from build123d import *

# Parameters (mm, degrees)
F0_W           = 127
F0_H           = 19.05
F1_DEPTH       = 88.9
F2_R           = 3.937
F2_R_2         = 2.413
F3_DEPTH       = 19.05
F5_D           = 6.35
F5_CBORE_D     = 11.176
F5_CBORE_DEPTH = 6.35
F7_DEPTH       = 19.051
F8_R           = 3.048


with BuildPart() as f1:
    # F0 (on Front) → F1 (new body)
    with BuildSketch(Plane.XZ):
        Rectangle(F0_W, F0_H)
    extrude(amount=-F1_DEPTH)

    # F2 (on face) → F3 (cut, through all)
    with BuildSketch(Plane.XY.offset(9.525)):
        with Locations((-53.975, 73.025)):
            Circle(F2_R)
        with Locations((-53.975, 9.525)):
            Circle(F2_R)
        with Locations((53.975, 9.525)):
            Circle(F2_R)
        with Locations((53.975, 73.025)):
            Circle(F2_R)
        with Locations((-6.35, 38.1)):
            Circle(F2_R_2)
        with Locations((12.7, 38.1)):
            Circle(F2_R_2)
        with Locations((12.7, 12.7)):
            Circle(F2_R_2)
        with Locations((-6.35, 12.7)):
            Circle(F2_R_2)
    extrude(amount=-F3_DEPTH, mode=Mode.SUBTRACT)

    # F5 (through all)
    with Locations(Plane(origin=(0, 0, -9.525), x_dir=(1, 0, 0), z_dir=(0, 0, -1))):
        with Locations((25.4, -69.85), (25.4, -44.45), (-41.275, -31.75), (-41.275, -6.35)):
            CounterBoreHole(F5_D / 2, F5_CBORE_D / 2, F5_CBORE_DEPTH)

    # F6 (on face) → F7 (cut, through all)
    with BuildSketch(Plane(origin=(0, 0, -9.525), x_dir=(1, 0, 0), z_dir=(0, 0, -1))):
        with BuildLine():
            ThreePointArc((63.5, -81.5884231275), (0, -88.9), (-63.5, -81.5884231275))
            Line((-63.5, -81.5884231275), (-63.5, -94.2089855671))
            Line((-63.5, -94.2089855671), (63.5, -94.2089855671))
            Line((63.5, -94.2089855671), (63.5, -81.5884231275))
        make_face()
    extrude(amount=-F7_DEPTH, mode=Mode.SUBTRACT)

    # F8
    f8_edges = [f1.edges().sort_by_distance(p)[0] for p in [
        (63.5, 81.588423, 0),
        (63.5, 0, 0),
        (-63.5, 81.588423, 0),
        (-63.5, 0, 0),
    ]]
    fillet(f8_edges, radius=F8_R)


solid = f1.part
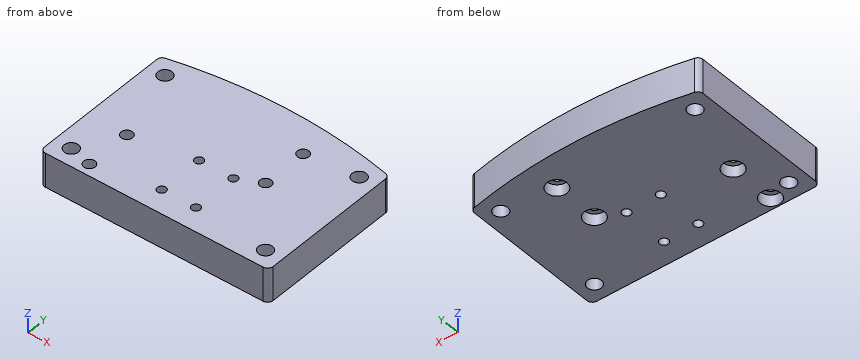
The listing builds one solid part. Answer for the finished solid, in the listing's coordinates (mm). Round coordinates to 2 decimals unless told otherwise and drop trailing zeros. Write each loop counter-clockwise with the first axis right and the second up, starting at its lowest first coordinate (ties: lowest second). Pieces come first, ordered by that corner, then holes. Notation, with made-up numbers: (87.25, -8) - (112.25, -8) arc R20 ccw to (112.25, -2) - close; hole circle Ø11 at (-29.75, 33.5). An arc over 180 degrees is marked (long way). Use one line per item in the form item = value. Start each with the question number.
Item 1: A cutting plane is placed at C-C (x = 12.7). Write down the section's boundary in (y, z) (3 decimals), plus the area to 3 significant figures.
Item 2: A cutting plane is placed at A-A (y = 31.75). Write down the section's boundary in (x, z) (3 decimals).
Item 3: Flat-ended cylindrical pins translate along their axes: pin 1 Ø7.5 at (x, y) = (25.4, 69.85) entering from -Z (3 decimals); pin 2 Ø2 at (x, z) = (22, 6) entering from +Y; pin 3 Ø3 at (x, z) = (50, 3.5) entering from +Y; pin 4 Ø13 at (x, y) = (25.4, 44.45) entering from +Z (3 decimals). Find the tip coordinate at first contact, or state that the pin passes through.
Item 4: A cutting plane is placed at B-B (z = -7.5). Give the number of separate pieces and of enclosed holes in the cut face, plus the area to 3 significant figures.
Item 5: Find the intervals of material crossed by line 1 (Y direction, x = 23.5, z = -3.5); line 2 (Y direction, x = -41, z = -1.25); line 3 (X direction, y = 8, z = 4), in increasing order. Write a range as [from, to].
The answers:
q1.outline = (0, -9.525) - (10.287, -9.525) - (10.287, 9.525) - (0, 9.525) - close; (15.113, -9.525) - (35.687, -9.525) - (35.687, 9.525) - (15.113, 9.525) - close; (40.513, -9.525) - (88.611, -9.525) - (88.611, 9.525) - (40.513, 9.525) - close
q1.area = 1,500 mm^2
q2.outline = (-63.5, -9.525) - (-46.863, -9.525) - (-46.863, -3.175) - (-44.45, -3.175) - (-44.45, 9.525) - (-63.5, 9.525) - close; (-38.1, -3.175) - (-35.687, -3.175) - (-35.687, -9.525) - (63.5, -9.525) - (63.5, 9.525) - (-38.1, 9.525) - close
q3.pin_1 = -3.175
q3.pin_2 = 88.11
q3.pin_3 = 84.66
q3.pin_4 = 9.525
q4.separate_pieces = 1
q4.enclosed_holes = 12
q4.area = 10,300 mm^2
q5.line_1 = [0, 39.19], [49.71, 64.59], [75.11, 87.91]
q5.line_2 = [0, 3.19], [9.51, 28.59], [34.91, 85.88]
q5.line_3 = [-63.5, -57.6], [-50.35, -43.99], [-38.56, 50.35], [57.6, 63.5]
